```python
from build123d import *

# Parameters (mm, degrees)
SKICA1_R                = 1.5
SKICA1_R_2              = 14.5
P_IDAT_VYSUNUT_M1_DEPTH = 10
SKICA2_R                = 8
P_IDAT_VYSUNUT_M2_DEPTH = 1


with BuildPart() as part:
    # Skica1 → Přidat vysunutím1 (new body)
    with BuildSketch(Plane.XY):
        with BuildLine():
            Line((-15, 12), (-15, 0))
            Line((-15, 0), (-15, -12))
            ThreePointArc((-15, -12), (-14.121320344, -14.121320344), (-12, -15))
            Line((-12, -15), (12, -15))
            ThreePointArc((12, -15), (14.121320344, -14.121320344), (15, -12))
            Line((15, -12), (15, 12))
            ThreePointArc((15, 12), (14.121320344, 14.121320344), (12, 15))
            Line((12, 15), (-12, 15))
            ThreePointArc((-12, 15), (-14.121320344, 14.121320344), (-15, 12))
        make_face()
        with Locations((-12, -12)):
            Circle(SKICA1_R, mode=Mode.SUBTRACT)
        with Locations((12, -12)):
            Circle(SKICA1_R, mode=Mode.SUBTRACT)
        with Locations((-12, 12)):
            Circle(SKICA1_R, mode=Mode.SUBTRACT)
        Circle(SKICA1_R_2, mode=Mode.SUBTRACT)
        with Locations((12, 12)):
            Circle(SKICA1_R, mode=Mode.SUBTRACT)
    extrude(amount=P_IDAT_VYSUNUT_M1_DEPTH)

    # Skica2 → Přidat vysunutím2 (add)
    with BuildSketch(Plane.XY):
        with BuildLine():
            ThreePointArc((-4.83465237, 6.373863542), (-4, 6.92820323), (-3.102601563, 7.373863542))
            Line((-3.102601563, 7.373863542), (-6.366712667, 13.027469816))
            ThreePointArc((-6.366712667, 13.027469816), (-7.25, 12.557368355), (-8.098763475, 12.027469816))
            Line((-8.098763475, 12.027469816), (-4.83465237, 6.373863542))
        make_face()
        Circle(SKICA2_R)
        with BuildLine():
            Line((14.465476141, 1), (7.937253933, 1))
            ThreePointArc((7.937253933, 1), (7.984298074, 0.5009833), (8, 0))
            ThreePointArc((8, 0), (7.984298074, -0.5009833), (7.937253933, -1))
            Line((7.937253933, -1), (14.465476141, -1))
            ThreePointArc((14.465476141, -1), (14.491366465, -0.500297885), (14.5, 0))
            ThreePointArc((14.5, 0), (14.491366465, 0.500297885), (14.465476141, 1))
        make_face()
        with BuildLine():
            Line((-6.366712667, -13.027469816), (-3.102601563, -7.373863542))
            ThreePointArc((-3.102601563, -7.373863542), (-4, -6.92820323), (-4.83465237, -6.373863542))
            Line((-4.83465237, -6.373863542), (-8.098763475, -12.027469816))
            ThreePointArc((-8.098763475, -12.027469816), (-7.25, -12.557368355), (-6.366712667, -13.027469816))
        make_face()
    extrude(amount=P_IDAT_VYSUNUT_M2_DEPTH)


solid = part.part
```
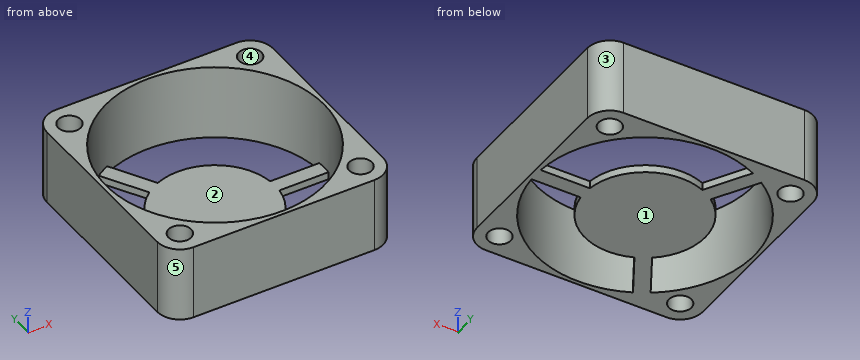
Design review of the part built by this model. Coordinates are the model's own, in mm. Face numbers are marked on the shaded views. A direction names the side the tool comes from. Give positions to 0.01 mm unless a question says otherwise; leave off trailing zeros. Write each loop counter-clockwise with the first axis right and the second up, starting at its lowest first coordinate (ties: lowest second). Pieces come first, ordered by that corner, then holes.
(1) Mouldability with a two-part tool opening along Y and no side actions: class the marked faces 3, 4 and 5 as +Y half, -Y half, draft (parallel to the pull), parting line (faces both ways), or undercut.
Checked values:
face 3: +Y half
face 4: undercut
face 5: -Y half
(2) Add section C-C (z = 3.5). Give the boundary of the cut face in (x, y).
Checked values:
outline: (-15, -12) arc R3 ccw to (-12, -15) - (12, -15) arc R3 ccw to (15, -12) - (15, 12) arc R3 ccw to (12, 15) - (-12, 15) arc R3 ccw to (-15, 12) - close; hole circle Ø29 at (0, 0); hole circle Ø3 at (-12, -12); hole circle Ø3 at (-12, 12); hole circle Ø3 at (12, -12); hole circle Ø3 at (12, 12)
(3) Wall thickness on line 1 along Y through (x, z) = (-12, 4); line 2 along Y through (x, z) = (-0.25, 4.25); line 3 along X through (y, z) = (-8.5, 9.25): over which ranges is each line inside the solid? List them lowest first.
Checked values:
line 1: y = -15 to -13.5, -10.5 to -8.14, 8.14 to 10.5, 13.5 to 15
line 2: y = -15 to -14.5, 14.5 to 15
line 3: x = -15 to -11.75, 11.75 to 15
(4) Add section B-B (y = 0). Give the boundary of the cut face in (x, z).
Checked values:
outline: (-15, 0) - (-14.5, 0) - (-14.5, 10) - (-15, 10) - close; (-8, 0) - (15, 0) - (15, 10) - (14.5, 10) - (14.5, 1) - (-8, 1) - close
(5) Clearance check with flat-ended pins moving along their axes: pin 1 Ø11.5 at (x, y) = (4, -1) entering from +Z; pin 2 Ø1.8 at (x, y) = (-12, 12) entering from +Z. State where each tip first meets the part, or that it passes through.
Checked values:
pin 1: stops at z = 1
pin 2: passes through
(6) Add section D-D (x = 0.5). Give the boundary of the cut face in (y, z).
Checked values:
outline: (-15, 0) - (-14.49, 0) - (-14.49, 10) - (-15, 10) - close; (-7.98, 0) - (7.98, 0) - (7.98, 1) - (-7.98, 1) - close; (14.49, 0) - (15, 0) - (15, 10) - (14.49, 10) - close
(7) Add section A-A (x = -10). Give the boundary of the cut face in (y, z), and give its area (3 significant figures).
Checked values:
outline: (-15, 0) - (-10.5, 0) - (-10.5, 10) - (-15, 10) - close; (10.5, 0) - (15, 0) - (15, 10) - (10.5, 10) - close
area: 90.0 mm2
(8) Tool access review of the marked faces 1 and 2: name each direction out of +Z, -Z, +X, -X, +Y, -Y from which nothing blocks a thin tool from reaching the whole face with its end or side.
Checked values:
face 1: -Z, +X, -X, +Y, -Y
face 2: +Z
